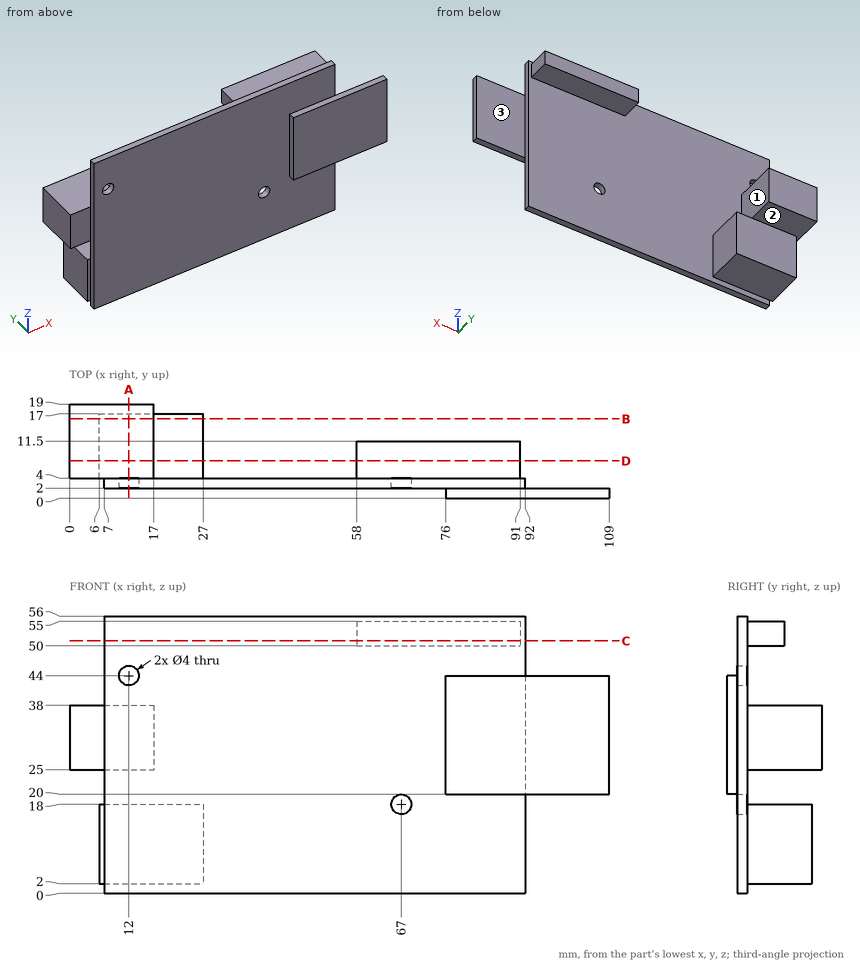
Job drawing, mm, ordinate dimensions from the low corner. One solid piece. A direction names the side the tool comes from. Give positions to 0.01 mm unless a question says otherwise; leave off trailing zeros. Loops run counter-clockwise (first coordinate to the right, second up) from the corner with the lowest first, then second, coordinate; pieces in that order, holes last. Notation, with made-up numbers: (-21, 56.25) -> (9, 56.25) arc R33 cw to (9, 87.25) -> close; hole circle Ø1 at (51.25, 23). An arc over 180 degrees is marked (long way). Write each question's results on one line, items separated by ' | '.
(1) Cut at D-D on y = 7.5. List the corners of the cut face in (x, z).
Geometry results:
outline: (0, 25) -> (17, 25) -> (17, 38) -> (0, 38) -> close; (6, 2) -> (27, 2) -> (27, 18) -> (6, 18) -> close; (58, 50) -> (91, 50) -> (91, 55) -> (58, 55) -> close
(2) Tool access for the marked faces 1, 2 and 3: list every direction of +Z, -Z, +X, -X, +Y, -Y with a clear straight run to the whole face (end or side of a thin tool).
Geometry results:
face 1: +Z, +X, +Y | face 2: +X, -X, +Y | face 3: +Z, -Z, +X, +Y
(3) Cut at A-A on x = 12. List the corners of the cut face in (y, z).
Geometry results:
outline: (2, 0) -> (4, 0) -> (4, 2) -> (17, 2) -> (17, 18) -> (4, 18) -> (4, 25) -> (19, 25) -> (19, 38) -> (4, 38) -> (4, 42) -> (2, 42) -> close; (2, 46) -> (4, 46) -> (4, 56) -> (2, 56) -> close
(4) Flat gauge pins, fed straight in: pin 1 Ø4.5 at (x, y) = (12, 12) entering from -Z; pin 2 Ø4 at (x, z) = (79.5, 53) entering from +Y; pin 3 Ø2 at (x, y) = (98, 1.5) entering from -Z; pin 4 Ø2.5 at (x, z) = (67, 18) entering from -Y. Where does each tip first touch, or does it go through?
Geometry results:
pin 1: stops at z = 2 | pin 2: stops at y = 11.5 | pin 3: stops at z = 20 | pin 4: passes through
(5) Cut at C-C on z = 51. List the corners of the cut face in (x, y), and give its area (4 significant figures).
Geometry results:
outline: (7, 2) -> (92, 2) -> (92, 4) -> (91, 4) -> (91, 11.5) -> (58, 11.5) -> (58, 4) -> (7, 4) -> close | area: 417.5 mm²
(6) Cut at B-B on y = 16. List the corners of the cut face in (x, z).
Geometry results:
outline: (0, 25) -> (17, 25) -> (17, 38) -> (0, 38) -> close; (6, 2) -> (27, 2) -> (27, 18) -> (6, 18) -> close
(7) Probe line 1 along Z through (x, y) = (12, 2.9); line 2 along X through (y, z) = (3, 18); line 3 along Z through (x, y) = (67, 3.2). List the from-to ranges inside material, lowest first.
Geometry results:
line 1: z = 0 to 42, 46 to 56 | line 2: x = 7 to 65, 69 to 92 | line 3: z = 0 to 16, 20 to 56
